Read the model definition and answer for the solid it produces. Units are mm, in the model's axes. A direction names the side the tool comes from. Round coordinates to 2 decimals unless told otherwise and drop trailing zeros. Order: outer loops, then holes, each group sorted by start corner. A loop starts at its lowest first (then second) coordinate and runs counter-clockwise, first axis right, second up. Notation, with made-up numbers: (-12, 1) -> (30, 1) arc R14 cw to (30, 20) -> close; hole circle Ø3 at (13.5, -13). An arc over 180 degrees is marked (long way). One line per item, written item: value. Start each with the question number.
1. Section C-C (y = 33) is taken. Give the vertices of the cut face in (x, z).
2. Consider line 1 (Z direction, x = -50, y = 3); line 2 (Z direction, x = -50, y = 9.25). Determine where each line is inside the solid, lowest interval first.
3. For faces 5 (the face through (1, 107, 1)), 6 (the face through (1, 5, 70)), determine the directions among +Z, -Z, +X, -X, +Y, -Y from which every point of the face is accessible in a straight line to the end or side of a thin tool.
4. Flat-ended cylindrical pins translate along their axes: pin 1 Ø10 at (x, z) = (-16.5, -49.5) entering from -Y; pin 2 Ø1.5 at (y, z) = (40.5, 29.5) entering from +X; pin 3 Ø3.5 at (x, z) = (50, 50) entering from +Y; pin 4 Ø6 at (x, y) = (-10, 97.5) entering from -Z. Find the tip coordinate at first contact, or state that the pin passes through.
5. Section A-A (z = 0) is taken. Give the vertices of the cut face in (x, y), then the cut area to 3 significant figures.
6. The mould has two halves that part along X. Classify faces 1 (the face through (-47.69, 61.84, -15.02)), 2 (the face through (-44.2, 110, -18.3)), 3 (the face through (-51.52, 2.96, 48.34)), 4 (the face through (52.4, 8, 46.8)): released by +X, released by -X, zero draft, split by the parting line, or undercut.
7. Section D-D (x = -61) is taken. Give the vertices of the cut face in (y, z), then the cut area to 3 significant figures.
8. Section B-B (x = 0) is taken. Give the vertices of the cut face in (y, z), then the cut area to 3 significant figures.
Autodesk Fusion 360 part; units mm, degrees
sketch "Sketch1" plane through (0, 0, 0) normal (0, 1, 0) x (1, 0, 0)
  line L0 (70, -70) -> (-70, -70)
  line L1 (-70, -70) -> (-70, 70)
  line L2 (-70, 70) -> (70, 70)
  line L3 (70, 70) -> (70, -70)
  line L4 (70, -70) -> (-70, 70) construction
  line L5 (-70, -70) -> (70, 70) construction
  dimension "d1" = 140
  dimension "d2" = 140
extrude "Extrude1" add sketch "Sketch1" along normal blind 10
sketch "Sketch2" plane through (0, 10, 0) normal (0, 1, 0) x (-1, 0, 0)
  line L0 (-70, -70) -> (70, -70)
  line L1 (70, -70) -> (70, 70)
  line L2 (70, 70) -> (-70, 70)
  line L3 (-70, 70) -> (-70, -70)
  circle A0 centre (0, 0) radius 50
  dimension "d5" = 100
extrude "Extrude2" add sketch "Sketch2" along normal blind 100 contours A0
sketch "Sketch3" plane through (0, 0, 0) normal (0, 0, 1) x (1, 0, 0)
  line L0 (-40, 80) -> (40, 80)
  line L1 (40, 80) -> (40, 40)
  line L2 (40, 40) -> (-40, 40)
  line L3 (-40, 40) -> (-40, 80)
  dimension "d8" = 80
  dimension "d9" = 40
  dimension "d10" = 40
  dimension "d11" = 40
sketch "Sketch4" plane through (0, 110, 0) normal (0, 1, 0) x (-1, 0, 0)
  circle A0 centre (0, 0) radius 50
  circle A1 centre (0, 0) radius 47.5
  dimension "d14" = 95
extrude "Extrude4" cut sketch "Sketch4" against normal blind 3 contours A1
sketch "Sketch5" plane through (0, 10, 0) normal (0, 1, 0) x (-1, 0, 0)
  circle A0 centre (0, 0) radius 50
  line L0 (-70, -70) -> (70, -70)
  line L1 (70, -70) -> (70, 70)
  line L2 (70, 70) -> (-70, 70)
  line L3 (-70, 70) -> (-70, -70)
  point P0 (50, -50)
  point P1 (-50, -50)
  point P2 (-50, 50)
  point P3 (50, 50)
  dimension "d17" = 20
  dimension "d18" = 20
  dimension "d19" = 20
  dimension "d20" = 20
  dimension "d21" = 20
  dimension "d22" = 20
  dimension "d23" = 20
  dimension "d24" = 20
hole "Hole1" at (50, 10, -50) at (-50, 10, -50) at (-50, 10, 50) at (50, 10, 50) direction (0, -1, 0) diameter 4.5 depth 40 tip angle 118 counterbore diameter 8 counterbore depth 4
fillet "Fillet1" radius 3 4 edges at (70, 5, 70) (-70, 5, 70) (70, 5, -70) (-70, 5, -70)
fillet "Fillet4" radius 5 1 edges at (46.6164, 10, 18.0808)
Answer:
1. outline: circle Ø100 at (0, 0)
2. line 1: -70 to -52.25, -47.75 to 47.75, 52.25 to 70
2. line 2: -70 to -54, -46 to 46, 54 to 70
3. face 5: +Y
3. face 6: +Z, +X, -X, +Y, -Y
4. pin 1: y = 0
4. pin 2: x = 40.91
4. pin 3: through
4. pin 4: z = -49.51
5. outline: (-70, 0) -> (70, 0) -> (70, 10) -> (55, 10) arc R5 cw to (50, 15) -> (50, 110) -> (47.5, 110) -> (47.5, 107) -> (-47.5, 107) -> (-47.5, 110) -> (-50, 110) -> (-50, 15) arc R5 cw to (-55, 10) -> (-70, 10) -> close
5. area: 11,100 mm^2
6. face 1: split by the parting line
6. face 2: zero draft
6. face 3: undercut
6. face 4: undercut
7. outline: (0, -70) -> (10, -70) -> (10, 70) -> (0, 70) -> close
7. area: 1,400 mm^2
8. outline: (0, -70) -> (10, -70) -> (10, -55) arc R5 cw to (15, -50) -> (110, -50) -> (110, -47.5) -> (107, -47.5) -> (107, 47.5) -> (110, 47.5) -> (110, 50) -> (15, 50) arc R5 cw to (10, 55) -> (10, 70) -> (0, 70) -> close
8. area: 11,100 mm^2
